Geometry check sheet. Reference: the model listing, model coordinates, mm. A direction names the side the tool comes from. Coordinates: 2 decimals unless noted, no trailing zeros. Loops run counter-clockwise (first coordinate to the right, second up) from the corner with the lowest first, then second, coordinate; pieces in that order, holes last. Notation, with made-up numbers: (54.25, 21.25) - (110.25, 21.25) arc R21 cw to (110.25, 39.25) - close; hole circle Ø8 at (8, 57.5). An arc over 180 degrees is marked (long way). One line per item, written item: value.
from build123d import *

# Parameters (mm, degrees)
SKETCH1_R           = 2.5
BOSS_EXTRUDE1_DEPTH = 10
SKETCH2_R           = 2.5
CUT_EXTRUDE1_DEPTH  = 10


with BuildPart() as part:
    # Sketch1 → Boss-Extrude1 (new body)
    with BuildSketch(Plane.XY):
        with BuildLine():
            Line((-190, -75), (190, -75))
            ThreePointArc((190, -75), (197.071067812, -72.071067812), (200, -65))
            Line((200, -65), (200, 65))
            ThreePointArc((200, 65), (197.071067812, 72.071067812), (190, 75))
            Line((190, 75), (-190, 75))
            ThreePointArc((-190, 75), (-197.071067812, 72.071067812), (-200, 65))
            Line((-200, 65), (-200, -65))
            ThreePointArc((-200, -65), (-197.071067812, -72.071067812), (-190, -75))
        make_face()
        with Locations((-190, 65)):
            Circle(SKETCH1_R, mode=Mode.SUBTRACT)
        with Locations(Location((-190, -65, 0), (0, 0, 180))):
            Circle(SKETCH1_R, mode=Mode.SUBTRACT)
        with Locations((190, -65)):
            Circle(SKETCH1_R, mode=Mode.SUBTRACT)
        with Locations(Location((190, 65, 0), (0, 0, 180))):
            Circle(SKETCH1_R, mode=Mode.SUBTRACT)
    extrude(amount=BOSS_EXTRUDE1_DEPTH)

    # Sketch2 → Cut-Extrude1 (cut)
    with BuildSketch(Plane.XY.offset(10)):
        Circle(SKETCH2_R)
        with BuildLine():
            Line((-60, -7.5), (-180, -7.5))
            ThreePointArc((-180, -7.5), (-187.5, 0), (-180, 7.5))
            Line((-180, 7.5), (-60, 7.5))
            ThreePointArc((-60, 7.5), (-52.5, 0), (-60, -7.5))
        make_face()
        with BuildLine():
            Line((60, -7.5), (180, -7.5))
            ThreePointArc((180, -7.5), (187.5, 0), (180, 7.5))
            Line((180, 7.5), (60, 7.5))
            ThreePointArc((60, 7.5), (52.5, 0), (60, -7.5))
        make_face()
    extrude(amount=-CUT_EXTRUDE1_DEPTH, mode=Mode.SUBTRACT)


solid = part.part
(1) Access from +Z, -Z, +X, -X, +Y, -Y to the whole of each face (thin tool, end or side, straight path). Record for faces 1 (the face through (-3, 1, 10)), 2 (the face through (119, -7.5, 5)).
Reply:
face 1: +Z, +X, -X, +Y, -Y
face 2: +Z, -Z
(2) Cross-section at B-B on x = 160. Record the cut outline in (y, z), and give its area (3 significant figures).
Reply:
outline: (-75, 0) - (-7.5, 0) - (-7.5, 10) - (-75, 10) - close; (7.5, 0) - (75, 0) - (75, 10) - (7.5, 10) - close
area: 1,350 mm2
(3) Material ranges on probe 1 along Y at (x, z) = (190, 7.5); probe 2 along Y at (x, z) = (-180.5, 2.5); probe 3 along Y at (x, z) = (0, 6.75), recorded low to high. Write a range as from..to.
Reply:
probe 1: -75..-67.5, -62.5..62.5, 67.5..75
probe 2: -75..-7.48, 7.48..75
probe 3: -75..-2.5, 2.5..75
(4) Go/stop test with a flat-tipped pin: pin 1 Ø4.5 at (x, y) = (-190, 65) entering from -Z. Record where the tip stops, or that it passes through.
Reply:
pin 1: through
(5) Cross-section at A-A on z = 8.25. Record the cut outline in (x, y).
Reply:
outline: (-200, -65) arc R10 ccw to (-190, -75) - (190, -75) arc R10 ccw to (200, -65) - (200, 65) arc R10 ccw to (190, 75) - (-190, 75) arc R10 ccw to (-200, 65) - close; hole circle Ø5 at (-190, -65); hole circle Ø5 at (-190, 65); hole (-180, -7.5) - (-60, -7.5) arc R7.5 ccw to (-60, 7.5) - (-180, 7.5) arc R7.5 ccw to start; hole circle Ø5 at (0, 0); hole (60, -7.5) - (180, -7.5) arc R7.5 ccw to (180, 7.5) - (60, 7.5) arc R7.5 ccw to start; hole circle Ø5 at (190, -65); hole circle Ø5 at (190, 65)
(6) Release check for a two-part mould opening along Y. For faces 3 (the face through (187.5, -0.16, 5.07)), 4 (the face through (-200, 1, 5)), 5 (the face through (-3, -75, 5)) record: pulls with the +Y half, pulls with the -Y half, needs draft (parallel to the pull), parting line crosses it, or undercut.
Reply:
face 3: undercut
face 4: needs draft
face 5: pulls with the -Y half
